Drawing for the job (mm, zero at the part's lowest x, y, z). Give positions to 0.01 mm unless a question says otherwise; leave off trailing zeros. Order: outer loops, then holes, each group sorted by start corner. A loop starts at its lowest first (then second) coordinate and runs counter-clockwise, first axis right, second up. Notation, with made-up numbers: (9, -19.5) - (40, -19.5) arc R16 cw to (40, 5.5) - close; hole circle Ø10 at (32, 82). An arc over 180 degrees is marked (long way). One line per item, written item: value.
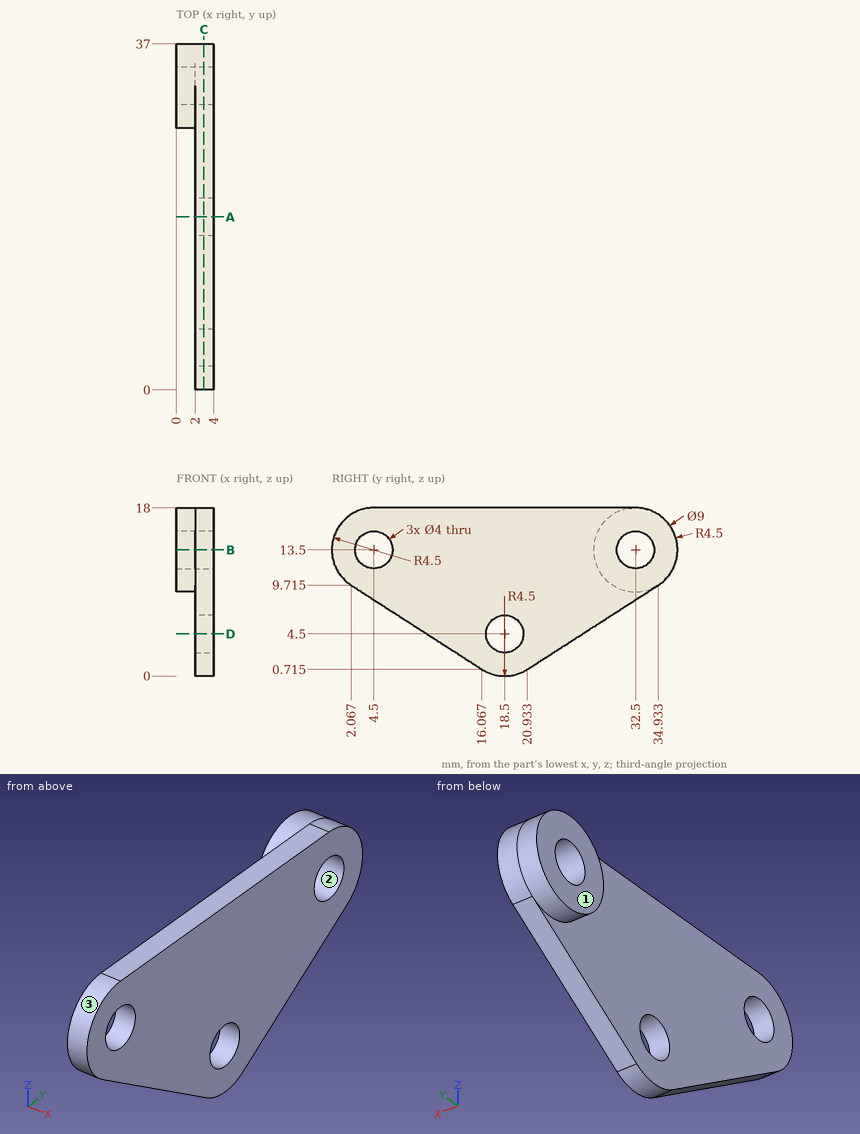
(1) Pull direction Z, two halves, no side cores. Call the marked faces 1, 2 and 3: +Z half, -Z half, draft (parallel to the pull), parting line (faces both ways), or undercut.
Completed:
face 1: draft
face 2: undercut
face 3: parting line
(2) Slice it at B-B, the plane z = 13.5. Give the cut face in (x, y).
Completed:
outline: (0, 28) - (2, 28) - (2, 6.5) - (4, 6.5) - (4, 30.5) - (0, 30.5) - close; (0, 34.5) - (4, 34.5) - (4, 37) - (0, 37) - close; (2, 0) - (4, 0) - (4, 2.5) - (2, 2.5) - close
(3) Slice it at D-D, the plane z = 4.5. Give the cut face in (x, y), and give its area (3 significant figures).
Completed:
outline: (2, 10.18) - (4, 10.18) - (4, 16.5) - (2, 16.5) - close; (2, 20.5) - (4, 20.5) - (4, 26.82) - (2, 26.82) - close
area: 25.3 mm²
(4) Slice it at C-C, the plane x = 2.95. Give the cut face in (y, z) (1 decimal).
Completed:
outline: (2.1, 9.7) - (16.1, 0.7) arc R4.5 ccw to (20.9, 0.7) - (34.9, 9.7) arc R4.5 ccw to (32.5, 18) - (4.5, 18) arc R4.5 ccw to start; hole circle Ø4 at (4.5, 13.5); hole circle Ø4 at (18.5, 4.5); hole circle Ø4 at (32.5, 13.5)
(5) Slice it at A-A, the plane y = 18.5. Give the cut face in (x, z), and give its area (3 significant figures).
Completed:
outline: (2, 0) - (4, 0) - (4, 2.5) - (2, 2.5) - close; (2, 6.5) - (4, 6.5) - (4, 18) - (2, 18) - close
area: 28.0 mm²
(6) Drill centre lines: line 1 (Y direction, x = 2.75, z = 13.5); line 2 (Z direction, x = 2.6, y = 18.5); line 3 (Y direction, x = 1.4, z = 13.5). Where is each one in solid material? Low to high.
Completed:
line 1: 0 to 2.5, 6.5 to 30.5, 34.5 to 37
line 2: 0 to 2.5, 6.5 to 18
line 3: 28 to 30.5, 34.5 to 37
(7) Pin check, flat tips, straight feed: P1, Ø3.5, axis at y = 32.5, z = 13.5, coming from the -X side; P2, Ø6.5, axis at y = 18.5, z = 4.5, coming from the -X side. Stop position of each tip, or through.
Completed:
P1: through
P2: x = 2
